For this review, take the finished solid that the model builds, in its own axes (mm). Face numbers are marked on the shaded views. A direction names the side the tool comes from. Coordinates: 2 decimals unless noted, no trailing zeros. Loops run counter-clockwise (first coordinate to the right, second up) from the corner with the lowest first, then second, coordinate; pieces in that order, holes last. Notation, with made-up numbers: (46, -2) -> (85, -2) arc R20 cw to (85, 30) -> close; hole circle Ø5 at (52, 17). An arc over 180 degrees is marked (long way). Use a Markdown table: item, result.
from build123d import *

# Parameters (mm, degrees)
ESQUISSE1_R             = 2
ESQUISSE1_R_2           = 1.75
BOSS_EXTRU_1_DEPTH      = 6
ENL_V_START             = -4
ESQUISSE2_R             = 2
ENL_V_MAT_EXTRU_1_DEPTH = 4
CHANFREIN2_SIZE         = 1.25


with BuildPart() as part:
    # Esquisse1 → Boss.-Extru.1 (new body)
    with BuildSketch(Plane.XY):
        with BuildLine():
            Line((0, 0), (17.5, 0))
            ThreePointArc((17.5, 0), (22.5, 5), (17.5, 10))
            Line((17.5, 10), (0, 10))
            ThreePointArc((0, 10), (-5, 5), (0, 0))
        make_face()
        with Locations((0, 5)):
            Circle(ESQUISSE1_R, mode=Mode.SUBTRACT)
        with Locations((17.5, 5)):
            Circle(ESQUISSE1_R_2, mode=Mode.SUBTRACT)
    extrude(amount=BOSS_EXTRU_1_DEPTH)

    # Esquisse2 → Enlèv. mat.-Extru.1 (cut)
    with BuildSketch(Plane.XY.offset(6).offset(ENL_V_START)):
        with BuildLine():
            Line((1.001951854, 8.872478855), (0, 9))
            ThreePointArc((0, 9), (-4, 5), (0, 1))
            Line((0, 1), (1.001951854, 1.127521145))
            Line((1.001951854, 1.127521145), (13.75, 2.75))
            ThreePointArc((13.75, 2.75), (15.07486756, 3.181421998), (15.891666667, 4.310243602))
            ThreePointArc((15.891666667, 4.310243602), (15.75, 5), (15.891666667, 5.689756398))
            ThreePointArc((15.891666667, 5.689756398), (15.07486756, 6.818578002), (13.75, 7.25))
            Line((13.75, 7.25), (1.001951854, 8.872478855))
        make_face()
        with Locations((0, 5)):
            Circle(ESQUISSE2_R, mode=Mode.SUBTRACT)
    extrude(amount=ENL_V_MAT_EXTRU_1_DEPTH, mode=Mode.SUBTRACT)

    # Chanfrein2
    chanfrein2_edges = [part.edges().sort_by_distance(p)[0] for p in [
        (15.75, 5, 0),
    ]]
    chamfer(chanfrein2_edges, length=CHANFREIN2_SIZE)


solid = part.part
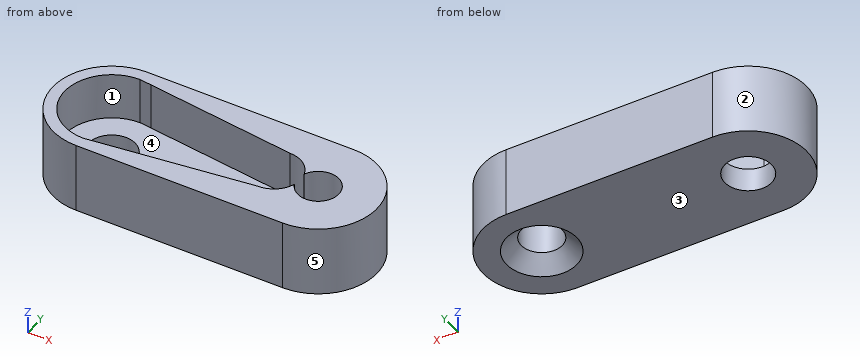
(1) Take a section at C-C on z = 0.8. Write out the cut boundary in (x, y).
Found:
| item | result |
|---|---|
| outline | (0, 0) -> (17.5, 0) arc R5 ccw to (17.5, 10) -> (0, 10) arc R5 ccw to start; hole circle Ø4 at (0, 5); hole circle Ø4.4 at (17.5, 5) |
(2) Mouldability with a two-part tool opening along Y and no side actions: class the marked faces 1, 2 and 3 as pulls with the +Y half, pulls with the -Y half, needs draft (parallel to the pull), parting line crosses it, or undercut.
Found:
| item | result |
|---|---|
| face 1 | undercut |
| face 2 | parting line crosses it |
| face 3 | needs draft |
(3) For line 1 along Y through (x, z) = (17.5, 5); line 2 along Y through (x, z) = (0, 1.55); line 3 along X through (y, z) = (5, 2.95), list the stretches that pass through material, from the lowest coordinate up.
Found:
| item | result |
|---|---|
| line 1 | y = 0 to 3.25, 6.75 to 10 |
| line 2 | y = 0 to 3, 7 to 10 |
| line 3 | x = -5 to -4, 19.25 to 22.5 |
(4) For pin 1 Ø1 at (x, y) = (-2, 5.5) entering from +Z; pin 2 Ø3.5 at (x, y) = (0, 5) entering from -Z; pin 3 Ø1.5 at (y, z) = (4, 3.5) entering from +X; pin 4 Ø5.5 at (x, y) = (17.5, 5) entering from -Z, all flat-tipped, find the tip position at first contact; note any pin that passes through.
Found:
| item | result |
|---|---|
| pin 1 | stops at z = 2 |
| pin 2 | passes through |
| pin 3 | stops at x = 22.49 |
| pin 4 | stops at z = 0.25 |
(5) Take a section at D-D on x = 5.25. Write out the cut boundary in (y, z), plus the area to 3 significant figures.
Found:
| item | result |
|---|---|
| outline | (0, 0) -> (10, 0) -> (10, 6) -> (8.33, 6) -> (8.33, 2) -> (1.67, 2) -> (1.67, 6) -> (0, 6) -> close |
| area | 33.3 mm^2 |
(6) Take a section at B-B on z = 5.15. Write out the cut boundary in (x, y), plus the area to 3 significant figures.
Found:
| item | result |
|---|---|
| outline | (0, 0) -> (17.5, 0) arc R5 ccw to (17.5, 10) -> (0, 10) arc R5 ccw to start; hole (0, 1) -> (13.75, 2.75) arc R2.25 ccw to (15.89, 4.31) arc R1.75 ccw (long way) to (15.89, 5.69) arc R2.25 ccw to (13.75, 7.25) -> (0, 9) arc R4 ccw to start |
| area | 125 mm^2 |
(7) Take a section at A-A on y = 5. Write out the cut boundary in (x, z).
Found:
| item | result |
|---|---|
| outline | (-5, 0) -> (-2, 0) -> (-2, 2) -> (-4, 2) -> (-4, 6) -> (-5, 6) -> close; (2, 0) -> (14.5, 0) -> (15.75, 1.25) -> (15.75, 2) -> (2, 2) -> close; (19.25, 1.25) -> (20.5, 0) -> (22.5, 0) -> (22.5, 6) -> (19.25, 6) -> close |
(8) For the marked faces 4 and 5, list the 3-axis set-ups (+Z, -Z, +X, -X, +Y, -Y) from which the entire face can be reached by the end or side of a thin tool; tool diameter is ignored.
Found:
| item | result |
|---|---|
| face 4 | +Z |
| face 5 | +Z, -Z, +X |
